Could you check a few things on this model? Use its own coordinates, in mm. A direction names the side the tool comes from. Coordinates: 2 decimals unless noted, no trailing zeros. Loops run counter-clockwise (first coordinate to the right, second up) from the corner with the lowest first, then second, coordinate; pieces in that order, holes last. Notation, with made-up numbers: (4, 72.25) -> (19, 72.25) arc R16 ccw to (19, 85.25) -> close; hole circle Ø11 at (-16, 27). An arc over 180 degrees is marked (long way). One line per question, with ' | ' between items. Start each with the question number.
(1) Suppose I cut it at A-A (y = -25). Please give me the cut outline in (x, z).
(2) Suppose I cut it at D-D (y = 10). Please give me the cut outline in (x, z).
(3) If I drill on line 1 along Z through (x, y) = (-46, 42.5); line 2 along Y through (x, z) = (25, 3.25); line 3 along X through (y, z) = (-25, 6.25), over which ranges is the centre line in solid material (lowest first)?
(4) If we mould it in two halves opening along Z, with no side actions, what happens to faces 5 (the face through (28, 5, 49)), 6 (the face through (-1, 1, 100)), 7 (the face through (47.15, 46.99, 94.93))? For each: pulls with the +Z half, pulls with the -Z half, needs draft (parallel to the pull), parting line crosses it, or undercut.
(5) Which directions (+Z, -Z, +X, -X, +Y, -Y) give clear straight access to the entire face, cutting with the end or side of a thin tool? Please do faces 1 (the face through (-27, 5, 49)), 2 (the face through (27, -27, 90)), 3 (the face through (-50, 3, 50)), 4 (the face through (-28, -27, 90)).
(6) Suppose I cut it at C-C (z = 80.5). Please give me the cut outline in (x, y), plus the area to 3 significant figures.
(7) I'm going to push flat-ended pins straight in: pin 1 Ø4 at (y, z) = (-15, 25) entering from -X; pin 2 Ø22.5 at (y, z) = (28.5, 68) entering from +X; pin 3 Ø1 at (x, z) = (-30.5, 13.5) entering from -Y. Where does each tip first touch, or does it pass through?
```python
from build123d import *

# Parameters (mm, degrees)
F1_DEPTH = 100
F2_W     = 100
F2_H     = 100
F3_DEPTH = 10
F4_W     = 45
F4_H     = 45
F5_DEPTH = 10
F6_R     = 10
F7_R     = 9
F8_DEPTH = 87


with BuildPart() as f1:
    # F0 (on Top) → F1 (new body)
    with BuildSketch(Plane.XY):
        Polygon((-5, -50), (0, -50), (5, -50), (5, -5), (50, -5), (50, 0), (50, 5), (5, 5), (5, 50), (0, 50), (-5, 50), (-5, 5), (-50, 5), (-50, 0), (-50, -5), (-5, -5), align=None)
    extrude(amount=F1_DEPTH)

    # F2 (on Top) → F3 (join)
    with BuildSketch(Plane.XY):
        Rectangle(F2_W, F2_H)
    extrude(amount=F3_DEPTH)

    # F4 (on face) → F5 (join)
    with BuildSketch(Plane.XY.offset(100)):
        with Locations((-27.5, 27.5)):
            Rectangle(F4_W, F4_H)
        Polygon((5, 50), (-5, 50), (-5, 5), (-50, 5), (-50, -5), (-5, -5), (-5, -50), (5, -50), (5, -5), (50, -5), (50, 5), (5, 5), align=None)
        with Locations((27.5, 27.5)):
            Rectangle(F4_W, F4_H)
        with Locations((27.5, -27.5)):
            Rectangle(F4_W, F4_H)
        with Locations((-27.5, -27.5)):
            Rectangle(F4_W, F4_H)
    extrude(amount=-F5_DEPTH)

    # F6
    f6_edges = [f1.edges().sort_by_distance(p)[0] for p in [
        (50, -50, 95),
        (50, -50, 5),
        (50, 50, 95),
        (50, 50, 5),
        (-50, -50, 95),
        (-50, -50, 5),
        (-50, 50, 95),
        (-50, 50, 5),
    ]]
    fillet(f6_edges, radius=F6_R)

    # F7 (on Top) → F8 (cut, symmetric)
    with BuildSketch(Plane.XY):
        with Locations((-25, -25)):
            Circle(F7_R)
        with Locations((25, 25)):
            Circle(F7_R)
    extrude(amount=F8_DEPTH, both=True, mode=Mode.SUBTRACT)


solid = f1.part
```
Checks:
1) outline: (-50, 0) -> (-34, 0) -> (-34, 10) -> (-50, 10) -> close; (-50, 90) -> (-5, 90) -> (-5, 10) -> (-16, 10) -> (-16, 0) -> (50, 0) -> (50, 10) -> (5, 10) -> (5, 90) -> (50, 90) -> (50, 100) -> (-50, 100) -> close
2) outline: (-50, 0) -> (50, 0) -> (50, 10) -> (5, 10) -> (5, 90) -> (50, 90) -> (50, 100) -> (-50, 100) -> (-50, 90) -> (-5, 90) -> (-5, 10) -> (-50, 10) -> close
3) line 1: z = 0 to 10, 90 to 100 | line 2: y = -50 to 16, 34 to 50 | line 3: x = -50 to -34, -16 to 50
4) face 5: undercut | face 6: pulls with the +Z half | face 7: needs draft
5) face 1: -X, +Y | face 2: +X, -Y | face 3: +Z, -Z, -X, +Y, -Y | face 4: -X, -Y
6) outline: (-50, -5) -> (-5, -5) -> (-5, -50) -> (5, -50) -> (5, -5) -> (50, -5) -> (50, 5) -> (5, 5) -> (5, 50) -> (-5, 50) -> (-5, 5) -> (-50, 5) -> close | area: 1,900 mm^2
7) pin 1: stops at x = -5 | pin 2: stops at x = 5 | pin 3: stops at y = -5
